Here's how the part is built. I have some questions about the finished solid (model axes, mm). A direction names the side the tool comes from. Round coordinates to 2 decimals unless told otherwise and drop trailing zeros. Write each loop counter-clockwise with the first axis right and the second up, starting at its lowest first coordinate (ties: lowest second). Pieces come first, ordered by that corner, then holes. Notation, with made-up numbers: (66.5, 71) - (110.5, 71) arc R32 cw to (110.5, 97) - close; hole circle Ø8 at (34.5, 44.25). An arc over 180 degrees is marked (long way). Return JSON: item names as keys, results as strings. Group by question number.
```python
from build123d import *

# Parameters (mm, degrees)
SKETCH1_R           = 12
BOSS_EXTRUDE1_DEPTH = 10
CHAMFER1_SIZE       = 3


with BuildPart() as part:
    # Sketch1 → Boss-Extrude1 (new body)
    with BuildSketch(Plane.XY):
        with BuildLine():
            Line((-35, 42), (-35, -42))
            Line((-35, -42), (-32, -45))
            Line((-32, -45), (-20, -45))
            Line((-20, -45), (-20, -33))
            ThreePointArc((-20, -33), (-15, -28), (-10, -33))
            Line((-10, -33), (-10, -45))
            Line((-10, -45), (5, -45))
            Line((5, -45), (19.965278914, -34.521198893))
            ThreePointArc((19.965278914, -34.521198893), (26.787044835, -31.157076231), (34.304689823, -30))
            Line((34.304689823, -30), (45, -30))
            Line((45, -30), (53, -22))
            Line((53, -22), (63, -22))
            Line((63, -22), (71, -30))
            Line((71, -30), (85, -30))
            Line((85, -30), (85, 30))
            Line((85, 30), (71, 30))
            Line((71, 30), (63, 22))
            Line((63, 22), (53, 22))
            Line((53, 22), (45, 30))
            Line((45, 30), (34.304689823, 30))
            ThreePointArc((34.304689823, 30), (26.787044835, 31.157076231), (19.965278914, 34.521198893))
            Line((19.965278914, 34.521198893), (5, 45))
            Line((5, 45), (-10, 45))
            Line((-10, 45), (-10, 33))
            ThreePointArc((-10, 33), (-15, 28), (-20, 33))
            Line((-20, 33), (-20, 45))
            Line((-20, 45), (-32, 45))
            Line((-32, 45), (-35, 42))
        make_face()
        Circle(SKETCH1_R, mode=Mode.SUBTRACT)
    extrude(amount=BOSS_EXTRUDE1_DEPTH)

    # Chamfer1
    chamfer1_edges = [part.edges().sort_by_distance(p)[0] for p in [
        (85, 30, 5),
        (85, -30, 5),
    ]]
    chamfer(chamfer1_edges, length=CHAMFER1_SIZE)


solid = part.part
```
1) Will these pins go through, and if not, where does the flat tip stop? pin 1 Ø4 at (x, z) = (31, 1.5) entering from +Y; pin 2 Ø5 at (x, z) = (63, 7.5) entering from +Y; pin 3 Ø3 at (y, z) = (36.5, 3) entering from +X; pin 4 Ø6 at (x, y) = (61.5, 6.5) entering from -Z.
2) I need wall thicknesses on line 1 along Y through (x, z) = (0, 5); line 2 along X through (y, z) = (29.5, 6.5); line 3 along X through (y, z) = (-23.5, 7.75). Which ranges of each line are inside material? Lowest first, please.
3) Imagine slicing it at C-C (x = 0). Please give me the cut outline in (y, z), plus the area to 3 significant figures.
4) For faces 4 (the flat face through (-34, -43, 5)), 5 (the flat face through (40, -30, 5)), 6 (the flat face through (67, -26, 5)), 7 (the flat face through (24, 1, 0)), 8 (the flat face through (49, 26, 5)), which set-ups out of +Z, -Z, +X, -X, +Y, -Y let a thin tool reach every point of the face, with its end or its side?
5) If we mould it in two halves opening along X, with no side actions, what happens to faces 1 (the flat face through (84, -28, 5)), 2 (the flat face through (40, 30, 5)), 3 (the cylindrical face through (-11.99, 0.53, 4.93))? For each: released by +X, released by -X, zero draft, split by the parting line, or undercut.
6) Imagine slicing it at A-A (y = 0). Please give me the cut outline in (x, z), plus the area to 3 significant figures.
7) Imagine slicing it at D-D (x = 76). Please give me the cut outline in (y, z), plus the area to 3 significant figures.
Results found:
{
 "1": {"pin 1": "stops at y = 30.57", "pin 2": "stops at y = 24.5", "pin 3": "stops at x = 19.28", "pin 4": "stops at z = 0"},
 "2": {"line 1": "y = -45 to -12, 12 to 45", "line 2": "x = -35 to -18.57, -11.43 to 45.5, 70.5 to 82.5", "line 3": "x = -35 to 51.5, 64.5 to 85"},
 "3": {"outline": "(-45, 0) - (-12, 0) - (-12, 10) - (-45, 10) - close; (12, 0) - (45, 0) - (45, 10) - (12, 10) - close", "area": "660 mm²"},
 "4": {"face 4": "+Z, -Z, -X, -Y", "face 5": "+Z, -Z, +X, -Y", "face 6": "+Z, -Z, -Y", "face 7": "-Z, +X, -X, +Y, -Y", "face 8": "+Z, -Z, +Y"},
 "5": {"face 1": "released by +X", "face 2": "zero draft", "face 3": "undercut"},
 "6": {"outline": "(-35, 0) - (-12, 0) - (-12, 10) - (-35, 10) - close; (12, 0) - (85, 0) - (85, 10) - (12, 10) - close", "area": "960 mm²"},
 "7": {"outline": "(-30, 0) - (30, 0) - (30, 10) - (-30, 10) - close", "area": "600 mm²"}
}
